Read the model definition and answer for the solid it produces. Units are mm, in the model's axes. Coordinates: 2 decimals unless noted, no trailing zeros. Loops run counter-clockwise (first coordinate to the right, second up) from the corner with the lowest first, then second, coordinate; pieces in that order, holes last. Notation, with made-up numbers: (-30, -33.75) - (29, -33.75) arc R15 ccw to (29, -12.75) - close; hole circle Ø11 at (-24, -19). An arc over 180 degrees is marked (long way). Use one line per item in the form item = value. Start each with the question number.
1) A cutting plane is placed at B-B (z = 2). Give the vertices of the cut face in (x, y).
2) A cutting plane is placed at A-A (x = 76.5). Give the vertices of the cut face in (y, z).
3) Consider line 1 (X direction, y = 30.5, z = 16.75); line 2 (Y direction, x = 42, z = 2.25); line 3 (X direction, y = 11, z = 23.25). Determine where each line is inside the solid, lowest interval first.
4) This flat-tipped pin is pushed along its axis until it touches: P1, Ø1.5, axis at x = 53.5, z = 21.5, coming from the -Y side. Where does it stop, or does it pass through?
from build123d import *

# Parameters (mm, degrees)
SKETCH1_W           = 135
SKETCH1_H           = 35
BOSS_EXTRUDE1_DEPTH = 26
FILLET1_R           = 5


with BuildPart() as part:
    # Sketch1 → Boss-Extrude1 (new body)
    with BuildSketch(Plane.XY):
        with Locations((67.5, 17.5)):
            Rectangle(SKETCH1_W, SKETCH1_H)
    extrude(amount=BOSS_EXTRUDE1_DEPTH)

    # Fillet1
    fillet1_edges = [part.edges().sort_by_distance(p)[0] for p in [
        (67.5, 35, 26),
        (0, 17.5, 26),
        (67.5, 0, 26),
        (0, 17.5, 0),
        (67.5, 35, 0),
        (135, 17.5, 0),
        (67.5, 0, 0),
        (135, 17.5, 26),
        (0, 0, 13),
        (0, 35, 13),
        (135, 35, 13),
        (135, 0, 13),
    ]]
    fillet(fillet1_edges, radius=FILLET1_R)


solid = part.part
Found:
q1.outline = (1, 5) arc R4 ccw to (5, 1) - (130, 1) arc R4 ccw to (134, 5) - (134, 30) arc R4 ccw to (130, 34) - (5, 34) arc R4 ccw to (1, 30) - close
q2.outline = (0, 5) arc R5 ccw to (5, 0) - (30, 0) arc R5 ccw to (35, 5) - (35, 21) arc R5 ccw to (30, 26) - (5, 26) arc R5 ccw to (0, 21) - close
q3.line_1 = 0.03 to 134.97
q3.line_2 = 0.82 to 34.18
q3.line_3 = 0.53 to 134.47
q4.P1 = 0
